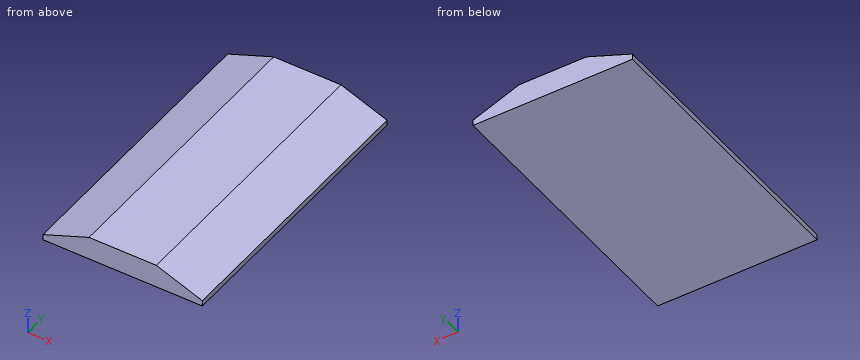
from build123d import *

# Parameters (mm, degrees)
F0_W     = 685.8
F0_H     = 1219.2
F1_DEPTH = 100.584
F2_SIZE2 = 76.2
F2_SIZE  = 198.12
F3_SIZE2 = 198.12
F3_SIZE  = 76.2


with BuildPart() as f1:
    # F0 (on Top) → F1 (new body)
    with BuildSketch(Plane.XY):
        with Locations((-19.1630474292, -94.6527993087)):
            Rectangle(F0_W, F0_H)
    extrude(amount=F1_DEPTH)

    # F2
    f2_edges = [f1.edges().sort_by_distance(p)[0] for p in [
        (-362.063047, -94.652799, 100.584),
    ]]
    f2_side = f1.faces().sort_by_distance((-19.163047, -94.652799, 100.584))[0]
    chamfer(f2_edges, length=F2_SIZE, length2=F2_SIZE2, reference=f2_side)

    # F3
    f3_edges = [f1.edges().sort_by_distance(p)[0] for p in [
        (323.736953, -94.652799, 100.584),
    ]]
    f3_side = f1.faces().sort_by_distance((323.736953, -94.652799, 50.292))[0]
    chamfer(f3_edges, length=F3_SIZE, length2=F3_SIZE2, reference=f3_side)


solid = f1.part
The listing builds one solid part. Answer for the finished solid, in the listing's coordinates (mm). Round coordinates to 2 decimals unless told otherwise and drop trailing zeros. Order: outer loops, then holes, each group sorted by start corner. A loop starts at its lowest first (then second) coordinate and runs counter-clockwise, first axis right, second up. Notation, with made-up numbers: M 68.5,7 L 119.5,7 A23 ccw 119.5,46 Z; hole C 40.5,31.5 d3. An arc over 180 degrees is marked long. Answer in a Markdown table with one row per item. Add a question column.
1) The part is cut by section B-B on z = 52.5. Determine the outline of the cut face in (x, y), plus the area to 3 significant figures.
2) The part is cut by section A-A on y = -598.5. Determine the outline of the cut face in (x, z).
3) The part is cut by section C-C on x = 183.5. Determine the outline of the cut face in (y, z), plus the area to 3 significant figures.
4) A flat-ended cylindrical pin translates along its axis: pin 1 Ø10 at (x, y) = (239, 241.5) entering from +Z. Find the tip coordinate at first contact, or state that the pin passes through.
5) Consider line 1 along Z through (x, y) = (157, 107.5); line 2 along Z through (x, y) = (-309, -12). Determine where each line is inside the solid, lowest interval first. Write a range as from..to.
Findings below:
| question | item | result |
|---|---|---|
| 1 | outline | M -288.96,-704.25 L 250.64,-704.25 L 250.64,514.95 L -288.96,514.95 Z |
| 1 | area | 658,000 mm² |
| 2 | outline | M -362.06,0 L 323.74,0 L 323.74,24.38 L 125.62,100.58 L -163.94,100.58 L -362.06,24.38 Z |
| 3 | outline | M -704.25,0 L 514.95,0 L 514.95,78.32 L -704.25,78.32 Z |
| 3 | area | 95,500 mm² |
| 4 | pin 1 | stops at z = 58.9 |
| 5 | line 1 | z = 0..88.51 |
| 5 | line 2 | z = 0..44.79 |
